Autodesk Inventor part; units mm, degrees
ref_plane "YZ Plane" through (0, 0, 0) normal (1, 0, 0) x (0, 1, 0)
ref_plane "XZ Plane" through (0, 0, 0) normal (0, 1, 0) x (-1, 0, 0)
ref_plane "XY Plane" through (0, 0, 0) normal (0, 0, 1) x (1, 0, 0)
sketch "Esquisse1" plane through (0, 0, 0) normal (0, 1, 0) x (-1, 0, 0)
  circle A0 centre (0, 0) radius 32.5
  dimension "d0" = 65
extrude "Extrusion1" add sketch "Esquisse1" along normal blind 1
sketch "Esquisse2" plane through (0, 1, 0) normal (0, 1, 0) x (1, 0, 0)
  circle A0 centre (0, 0) radius 32.5
  circle A1 centre (0, 0) radius 3
  dimension "d3" = 6
extrude "Extrusion2" cut sketch "Esquisse2" against normal through all contours A1
sketch "Esquisse3" plane through (0, 1, 0) normal (0, 1, 0) x (1, 0, 0)
  circle A0 centre (0, 0) radius 3
  circle A1 centre (0, 0) radius 32.5
  line L0 (0, 0) -> (0, 32.5) construction
  circle A2 centre (0, 27) radius 1.5
  circle A3 centre (-23.3827, 13.5) radius 1.5
  circle A4 centre (-23.3827, -13.5) radius 1.5
  circle A5 centre (0, -27) radius 1.5
  circle A6 centre (23.3827, -13.5) radius 1.5
  circle A7 centre (23.3827, 13.5) radius 1.5
  dimension "d6" = 27
  dimension "d7" = 3
  dimension "d10" = 360
extrude "Extrusion3" cut sketch "Esquisse3" against normal through all contours A2 | A3 | A4 | A5 | A6 | A7
properties part number "wheel_adapter"
Geometry check sheet. Reference: the model listing, model coordinates, mm. Give positions to 0.01 mm unless a question says otherwise; leave off trailing zeros. Write each loop counter-clockwise with the first axis right and the second up, starting at its lowest first coordinate (ties: lowest second). Pieces come first, ordered by that corner, then holes. Notation, with made-up numbers: M 19.5,-32 L 62.5,-32 A24 ccw 62.5,-2 Z; hole C 83,73 d8. An arc over 180 degrees is marked long. Answer as CSV lines item,"result". Start each with the question number.
Q1. Section check D-D, the plane z = -13.5. Record the cut outline in (x, y).
Q2. Section check C-C, the plane z = 1. Record the cut outline in (x, y), then the cut area to 3 significant figures.
Q3. Section check B-B, the plane y = 0.2. Record the cut outline in (x, z).
Q4. Section check A-A, the plane x = 0. Record the cut outline in (y, z).
Q5. Material ranges on L1, parallel to Z at x = 0, y = 0.25; L2, parallel to X at y = 0.8, z = 13.5; L3, parallel to X at y = 0.7, z = -27, recorded low to high.
Q6. Go/stop test with a flat-tipped pin: pin 1 (3.5 mm diameter, centred on x = 0, z = 0, fed in from -Y). Record where the tip stops, or that it passes through.
Q7. Release check for a two-part mould opening along X. For faces 1 (the face through (-0.195, 0.507, -28.487)), 2 (the face through (-7, 0, 0)), 3 (the face through (-31, 0.49, -9.76)) record: pulls with the +X half, pulls with the -X half, needs draft (parallel to the pull), parting line crosses it, or undercut.
Geometry says:
1,outline,"M -29.56,0 L -24.88,0 L -24.88,1 L -29.56,1 Z; M -21.88,0 L 21.88,0 L 21.88,1 L -21.88,1 Z; M 24.88,0 L 29.56,0 L 29.56,1 L 24.88,1 Z"
2,outline,"M -32.48,0 L -2.83,0 L -2.83,1 L -32.48,1 Z; M 2.83,0 L 32.48,0 L 32.48,1 L 2.83,1 Z"
2,area,"59.3 mm^2"
3,outline,"C 0,0 d65; hole C -23.38,-13.5 d3; hole C -23.38,13.5 d3; hole C 0,0 d6; hole C 0,-27 d3; hole C 0,27 d3; hole C 23.38,-13.5 d3; hole C 23.38,13.5 d3"
4,outline,"M 0,-32.5 L 1,-32.5 L 1,-28.5 L 0,-28.5 Z; M 0,-25.5 L 1,-25.5 L 1,-3 L 0,-3 Z; M 0,3 L 1,3 L 1,25.5 L 0,25.5 Z; M 0,28.5 L 1,28.5 L 1,32.5 L 0,32.5 Z"
5,L1,"-32.5 to -28.5, -25.5 to -3, 3 to 25.5, 28.5 to 32.5"
5,L2,"-29.56 to -24.88, -21.88 to 21.88, 24.88 to 29.56"
5,L3,"-18.09 to -1.5, 1.5 to 18.09"
6,pin 1,"through"
7,face 1,"undercut"
7,face 2,"needs draft"
7,face 3,"parting line crosses it"
